The listing builds one solid part. Answer for the finished solid, in the listing's coordinates (mm). A direction names the side the tool comes from. Give positions to 0.01 mm unless a question says otherwise; leave off trailing zeros. Write each loop counter-clockwise with the first axis right and the second up, starting at its lowest first coordinate (ties: lowest second). Pieces come first, ordered by that corner, then holes. Notation, with made-up numbers: (64.5, -1) - (89.5, -1) arc R22 ccw to (89.5, 10) - close; hole circle Ø7 at (24.5, 17). An arc over 180 degrees is marked (long way). Return JSON: item names as keys, results as strings.
from build123d import *

# Parameters (mm, degrees)
CROQUIS1_W                                  = 115
CROQUIS1_H                                  = 70
SALIENTE_EXTRUIR1_DEPTH                     = 5
SALIENTE_EXTRUIR2_DEPTH                     = 55
CROQUIS3_W                                  = 60
CROQUIS3_H                                  = 5
SALIENTE_EXTRUIR3_DEPTH                     = 110
CROQUIS4_W                                  = 15
CROQUIS4_H                                  = 15
SALIENTE_EXTRUIR4_DEPTH                     = 5
REFRENTADO_PARA_TORNILLO_CON_CABEZA_2_COUNT = 2
REFRENTADO_PARA_TORNILLO_CON_CABEZA_2_PITCH = 45


with BuildPart() as part:
    # Croquis1 → Saliente-Extruir1 (new body)
    with BuildSketch(Plane(origin=(0, 0, 0), x_dir=(1, 0, 0), z_dir=(0, 1, 0))):
        with Locations((57.5, 35)):
            Rectangle(CROQUIS1_W, CROQUIS1_H)
    extrude(amount=SALIENTE_EXTRUIR1_DEPTH)

    # Croquis2 → Saliente-Extruir2 (add)
    with BuildSketch(Plane(origin=(0, 5, 0), x_dir=(1, 0, 0), z_dir=(0, 1, 0))):
        Polygon((0, 0), (115, 0), (115, 70), (0, 70), (0, 65), (110, 65), (110, 5), (0, 5), align=None)
    extrude(amount=SALIENTE_EXTRUIR2_DEPTH)

    # Croquis3 → Saliente-Extruir3 (add)
    with BuildSketch(Plane.ZY.offset(-110)):
        with Locations((-35, 57.5)):
            Rectangle(CROQUIS3_W, CROQUIS3_H)
    extrude(amount=SALIENTE_EXTRUIR3_DEPTH)

    # Croquis4 → Saliente-Extruir4 (add)
    with BuildSketch(Plane.ZY.offset(-110)):
        with Locations((-57.5, 17.5)):
            Rectangle(CROQUIS4_W, CROQUIS4_H)
        with Locations((-12.5, 17.5)):
            Rectangle(CROQUIS4_W, CROQUIS4_H)
    extrude(amount=SALIENTE_EXTRUIR4_DEPTH)

    # Croquis7 → Refrentado para tornillo con cabeza hueca de M41 (revolve, cut)
    with BuildSketch(Plane(origin=(115, 17.5, -12.5), x_dir=(0, 0, -1), z_dir=(0, 1, 0))):
        Polygon((0, 0), (0, 21.851936393), (2.25, 20.5), (2.25, 3.2), (4, 3.2), (4, 0.025), (4.025, 0), align=None)
    refrentado_para_tornillo_con_cabeza_huec = revolve(axis=Axis((121.35, 17.5, -12.5), (-1, 0, 0)), mode=Mode.SUBTRACT)

    # Refrentado para tornillo con cabeza  2: Refrentado para tornillo con cabeza hueca de M41 ×2
    with Locations(*[(0, 0, -i * REFRENTADO_PARA_TORNILLO_CON_CABEZA_2_PITCH) for i in range(1, REFRENTADO_PARA_TORNILLO_CON_CABEZA_2_COUNT)]):
        add(refrentado_para_tornillo_con_cabeza_huec, mode=Mode.SUBTRACT)


solid = part.part
Item 1: A cutting plane is placed at A-A on z = -12.5. Determine the outline of the cut face in (x, y) (3 decimals).
Answer below:
{"outline": "(0, 0) - (115, 0) - (115, 13.475) - (114.975, 13.5) - (111.8, 13.5) - (111.8, 15.25) - (105, 15.25) - (105, 10) - (110, 10) - (110, 5) - (0, 5) - close; (0, 55) - (110, 55) - (110, 25) - (105, 25) - (105, 19.75) - (111.8, 19.75) - (111.8, 21.5) - (114.975, 21.5) - (115, 21.525) - (115, 60) - (0, 60) - close"}
Item 2: Consider L1, parallel to Z at x = 107.5, y = 17.5; L2, parallel to Z at x = 114.1, y = 17.5; L3, parallel to Y at x = 108, z = -12.5. Determine where each line is inside the solid, lowest interval first.
Answer below:
{"L1": "z = -70 to -59.75, -55.25 to -50, -20 to -14.75, -10.25 to 0", "L2": "z = -70 to -61.5, -53.5 to -16.5, -8.5 to 0", "L3": "y = 0 to 5, 10 to 15.25, 19.75 to 25, 55 to 60"}
Item 3: For faces 5 (the face through (113.41, 16.299, -61.315)), 6 (the face through (57, 0, -35)), 7 (the face through (108, 17, -50)), determine the directions among +Z, -Z, +X, -X, +Y, -Y from which every point of the face is accessible in a straight line to the end or side of a thin tool.
Answer below:
{"face 5": "+X", "face 6": "+Z, -Z, +X, -X, -Y", "face 7": "-X"}
Item 4: A cutting plane is placed at D-D on y = 17.5. Give the number of separate pieces and of enclosed holes in the cut face, then the cut area to 3 significant figures.
Answer below:
{"separate pieces": "3", "enclosed holes": "0", "area": "1,490 mm²"}
Item 5: A cutting plane is placed at C-C on y = 36. Determine the outline of the cut face in (x, z).
Answer below:
{"outline": "(0, -70) - (115, -70) - (115, 0) - (0, 0) - (0, -5) - (110, -5) - (110, -65) - (0, -65) - close"}
Item 6: The mould has two halves that part along Z. Classify faces 1 (the face through (58, 30, -70)), 2 (the face through (115, 30, -35)), 3 (the face through (54, 5, -35)), 4 (the face through (108, 25, -13)): +Z half, -Z half, draft (parallel to the pull), parting line (faces both ways), or undercut.
Answer below:
{"face 1": "-Z half", "face 2": "draft", "face 3": "undercut", "face 4": "undercut"}
Item 7: A cutting plane is placed at B-B on x = 87. Determine the outline of the cut face in (y, z), then the cut area to 3 significant figures.
Answer below:
{"outline": "(0, -70) - (60, -70) - (60, 0) - (0, 0) - close; hole (5, -65) - (55, -65) - (55, -5) - (5, -5) - close", "area": "1,200 mm²"}
Item 8: Flat-ended cylindrical pins translate along their axes: P1, Ø6, axis at y = 17.5, z = -12.5, coming from the +X side; P2, Ø6.5, axis at y = 17.5, z = -12.5, coming from the -X side; P3, Ø1, axis at y = 12.5, z = -24, coming from the -X side. Find the tip coordinate at first contact, or state that the pin passes through.
Answer below:
{"P1": "stops at x = 111.8", "P2": "stops at x = 105", "P3": "stops at x = 110"}
